Could you check a few things on this model? Use its own coordinates, in mm. A direction names the side the tool comes from. Give positions to 0.01 mm unless a question says otherwise; leave off trailing zeros. Order: outer loops, then holes, each group sorted by start corner. A loop starts at its lowest first (then second) coordinate and runs counter-clockwise, first axis right, second up. Notation, with made-up numbers: (31.25, -18.75) - (35.25, -18.75) arc R35 ccw to (35.25, 14.25) - close; hole circle Ø5 at (-13, -21). An arc over 180 degrees is marked (long way). Put each result on its own line as item: value.
from build123d import *

# Parameters (mm, degrees)
SKETCH1_W            = 110
SKETCH1_H            = 80
BOSS_EXTRUDE1_DEPTH  = 25
SKETCH2_R            = 4.75
CUT_EXTRUDE1_DEPTH   = 25
LPATTERN1_COUNT      = 2
LPATTERN1_PITCH      = 85
LPATTERN1_COUNT_DIR2 = 2
LPATTERN1_PITCH_DIR2 = 61.8
SKETCH3_R            = 35
BOSS_EXTRUDE2_DEPTH  = 50
SKETCH4_R            = 37.75
BOSS_EXTRUDE3_DEPTH  = 50
SKETCH5_R            = 28.5
CUT_EXTRUDE2_DEPTH   = 75
SKETCH6_R            = 23
CUT_EXTRUDE3_DEPTH   = 50
FILLET1_R            = 2


with BuildPart() as part:
    # Sketch1 → Boss-Extrude1 (new body)
    with BuildSketch(Plane.XY):
        Rectangle(SKETCH1_W, SKETCH1_H)
    extrude(amount=BOSS_EXTRUDE1_DEPTH)

    # Sketch2 → Cut-Extrude1 (cut)
    with BuildSketch(Plane.XY.offset(25)):
        with Locations((-42.5, -30.9)):
            Circle(SKETCH2_R)
    cut_extrude1 = extrude(amount=-CUT_EXTRUDE1_DEPTH, mode=Mode.SUBTRACT)

    # LPattern1: Cut-Extrude1 2 × 2
    with Locations(*[(i * LPATTERN1_PITCH, j * LPATTERN1_PITCH_DIR2, 0) for i in range(LPATTERN1_COUNT) for j in range(LPATTERN1_COUNT_DIR2) if (i, j) != (0, 0)]):
        add(cut_extrude1, mode=Mode.SUBTRACT)

    # Sketch3 → Boss-Extrude2 (add)
    with BuildSketch(Plane.XY.offset(25)):
        Circle(SKETCH3_R)
    extrude(amount=BOSS_EXTRUDE2_DEPTH)

    # Sketch4 → Boss-Extrude3 (add)
    with BuildSketch(Plane(origin=(0, 0, 0), x_dir=(-1, 0, 0), z_dir=(0, 0, -1))):
        Circle(SKETCH4_R)
    extrude(amount=BOSS_EXTRUDE3_DEPTH)

    # Sketch5 → Cut-Extrude2 (cut)
    with BuildSketch(Plane.XY.offset(75)):
        Circle(SKETCH5_R)
    extrude(amount=-CUT_EXTRUDE2_DEPTH, mode=Mode.SUBTRACT)

    # Sketch6 → Cut-Extrude3 (cut)
    with BuildSketch(Plane.XY):
        Circle(SKETCH6_R)
    extrude(amount=-CUT_EXTRUDE3_DEPTH, mode=Mode.SUBTRACT)

    # Fillet1
    fillet1_edges = [part.edges().sort_by_distance(p)[0] for p in [
        (-55, 0, 25),
        (0, -40, 25),
        (-35, 0, 75),
        (55, 0, 25),
        (55, -40, 12.5),
        (-55, -40, 12.5),
        (-55, 40, 12.5),
        (55, 40, 12.5),
        (0, 40, 25),
    ]]
    fillet(fillet1_edges, radius=FILLET1_R)


solid = part.part
1) Suppose I cut it at B-B, the plane z = 10. List the corners of the cut face in (x, y) for me.
Filled in:
outline: (-55, -38) arc R2 ccw to (-53, -40) - (53, -40) arc R2 ccw to (55, -38) - (55, 38) arc R2 ccw to (53, 40) - (-53, 40) arc R2 ccw to (-55, 38) - close; hole circle Ø9.5 at (-42.5, -30.9); hole circle Ø9.5 at (-42.5, 30.9); hole circle Ø57 at (0, 0); hole circle Ø9.5 at (42.5, -30.9); hole circle Ø9.5 at (42.5, 30.9)
2) Suppose I cut it at A-A, the plane x = -42.5. List the corners of the cut face in (y, z) for me, and give its area (3 significant figures).
Filled in:
outline: (-40, 0) - (-35.65, 0) - (-35.65, 25) - (-38, 25) arc R2 ccw to (-40, 23) - close; (-26.15, 0) - (26.15, 0) - (26.15, 25) - (-26.15, 25) - close; (35.65, 0) - (40, 0) - (40, 23) arc R2 ccw to (38, 25) - (35.65, 25) - close
area: 1,520 mm^2
3) We'd pull the mould along Y, two halves only. Please class faces 1 (the flat face through (-1, 40, 11)), 2 (the cylindrical face through (-28, -21, 49)), 3 (the cylindrical face through (26.327, -10.916, 38.025)): pulls with the +Y half, pulls with the -Y half, needs draft (parallel to the pull), parting line crosses it, or undercut.
Filled in:
face 1: pulls with the +Y half
face 2: parting line crosses it
face 3: undercut
4) Suppose I cut it at C-C, the plane x = 0. List the corners of the cut face in (y, z) for me.
Filled in:
outline: (-40, 0) - (-37.75, 0) - (-37.75, -50) - (-23, -50) - (-23, 0) - (-28.5, 0) - (-28.5, 75) - (-33, 75) arc R2 ccw to (-35, 73) - (-35, 25) - (-38, 25) arc R2 ccw to (-40, 23) - close; (23, -50) - (37.75, -50) - (37.75, 0) - (40, 0) - (40, 23) arc R2 ccw to (38, 25) - (35, 25) - (35, 73) arc R2 ccw to (33, 75) - (28.5, 75) - (28.5, 0) - (23, 0) - close
5) I'm going to push flat-ended pins straight in: pin 1 (10 mm diameter, centred on y = 17.5, z = -11, fed in from +X); pin 2 (4 mm diameter, centred on x = 21, z = 56, fed in from -Y); pin 3 (2 mm diameter, centred on x = -25.5, z = -36.5, fed in from +Y). Where does each tip first touch, or does it pass through?
Filled in:
pin 1: stops at x = 35.62
pin 2: stops at y = -29.39
pin 3: stops at y = 28.72
6) If I drill on line 1 (Y direction, x = 42.5, z = 15); line 2 (Z direction, x = -48.5, y = -11.5); line 3 (X direction, y = 4, z = 19.5), over which ranges is the centre line in solid material (lowest first)? Write a range as [from, to].
Filled in:
line 1: y = [-40, -35.65], [-26.15, 26.15], [35.65, 40]
line 2: z = [0, 25]
line 3: x = [-55, -28.22], [28.22, 55]
7) Suppose I cut it at D-D, the plane z = -28. List the corners of the cut face in (x, y) for me.
Filled in:
outline: circle Ø75.5 at (0, 0); hole circle Ø46 at (0, 0)
8) Which directions (+Z, -Z, +X, -X, +Y, -Y) give clear straight access to the entire face, cutting with the end or side of a thin tool? Please do faces 4 (the cylindrical face through (-36.007, 11.339, -24.65)), 5 (the flat face through (-55, -1, 11)), 6 (the flat face through (2, 23.4, 0)).
Filled in:
face 4: -Z
face 5: +Z, -Z, -X, +Y, -Y
face 6: +Z
